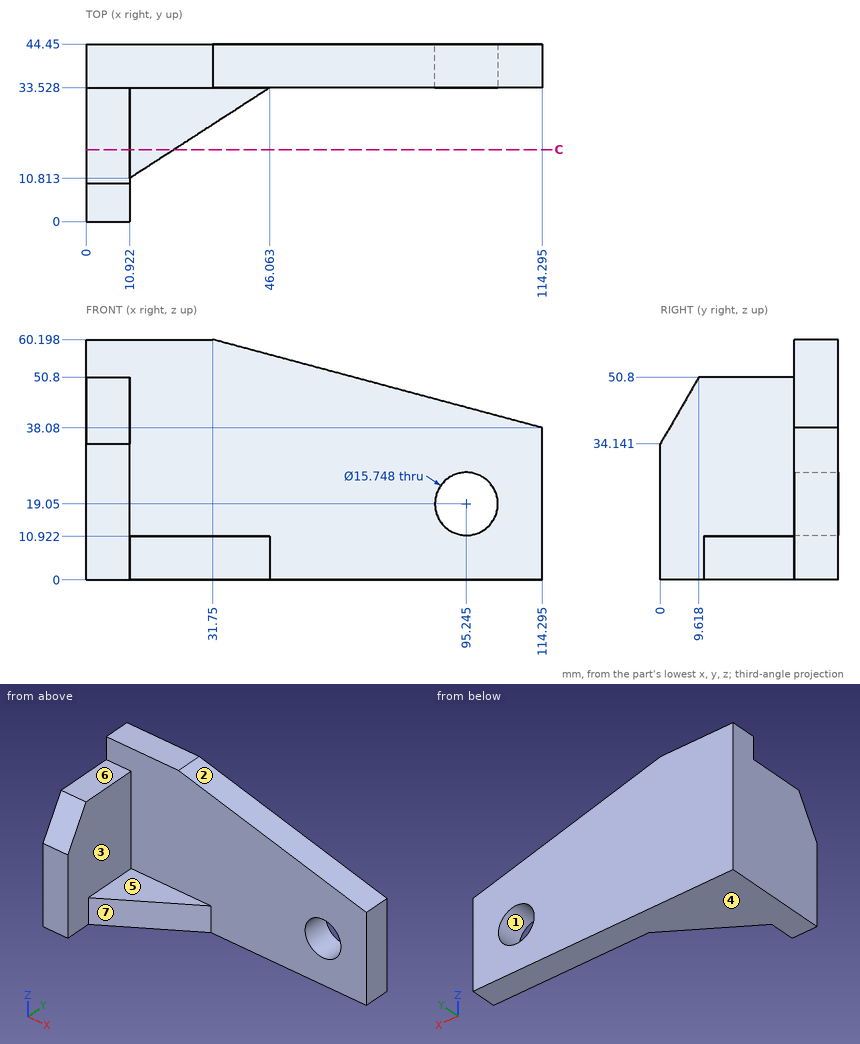
Here's the drawing with two shaded views (mm, measured from the low corner). I have some questions. A direction names the side the tool comes from. Give positions to 0.01 mm unless a question says otherwise; leave off trailing zeros. Order: outer loops, then holes, each group sorted by start corner. A loop starts at its lowest first (then second) coordinate and runs counter-clockwise, first axis right, second up. Notation, with made-up numbers: (79, -37.75) -> (90, -37.75) arc R36 ccw to (90, -2.75) -> close; hole circle Ø10 at (46, 69.5). An arc over 180 degrees is marked (long way). Use a Markdown table: item, result. Add a question column.
Item 1: Will these pins go through, and if not, where does the flat tip stop? pin 1 (9.5 mm diameter, centred on x = 95.24, z = 19.05, fed in from -Y); pin 2 (17 mm diameter, centred on y = 15.5, z = 20, fed in from +X); pin 3 (1.5 mm diameter, centred on x = 40, z = 27, fed in from -Y); pin 4 (8.5 mm diameter, centred on x = 7.5, y = 17, fed in from +Z).
Item 2: For the marked faces 5, 6 and 7, which set-ups out of +Z, -Z, +X, -X, +Y, -Y let a thin tool reach every point of the face, with its end or its side?
Item 3: I need wall thicknesses on line 1 (X direction, y = 39, z = 19) (1 decimal); line 2 (Z direction, x = 24.5, y = 26.5). Which ranges of each line are inside material? Lowest first, please.
Item 4: If we mould it in two halves opening along Z, with no side actions, what happens to the marked faces 1, 2, 3 and 4? For each: pulls with the +Z half, pulls with the -Z half, needs draft (parallel to the pull), parting line crosses it, or undercut.
Item 5: Imagine slicing it at C-C on y = 18. Please give me the cut outline in (x, z), plus the area to 3 significant figures.
Data:
| question | item | result |
|---|---|---|
| 1 | pin 1 | passes through |
| 1 | pin 2 | stops at x = 10.92 |
| 1 | pin 3 | stops at y = 33.53 |
| 1 | pin 4 | stops at z = 50.8 |
| 2 | face 5 | +Z, +X, -Y |
| 2 | face 6 | +Z, +X, -X, -Y |
| 2 | face 7 | +Z, -Z, +X, -Y |
| 3 | line 1 | x = 0 to 87.4, 103.1 to 114.3 |
| 3 | line 2 | z = 0 to 10.92 |
| 4 | face 1 | undercut |
| 4 | face 2 | pulls with the +Z half |
| 4 | face 3 | needs draft |
| 4 | face 4 | pulls with the -Z half |
| 5 | outline | (0, 0) -> (22.04, 0) -> (22.04, 10.92) -> (10.92, 10.92) -> (10.92, 50.8) -> (0, 50.8) -> close |
| 5 | area | 676 mm² |
